from build123d import *

# Parameters (mm, degrees)
SKETCH1_R           = 4.6
SKETCH1_R_2         = 3
BOSS_EXTRUDE1_DEPTH = 6.6
SKETCH2_R           = 4.1
BOSS_EXTRUDE2_DEPTH = 6
CHAMFER2_SIZE       = 0.5
CHAMFER3_SIZE       = 0.4
CHAMFER4_SIZE       = 0.4
CHAMFER4_SIZE2      = 0.8
CHAMFER5_SIZE       = 0.4


with BuildPart() as part:
    # Sketch1 → Boss-Extrude1 (new body)
    with BuildSketch(Plane.XY):
        Circle(SKETCH1_R)
        Circle(SKETCH1_R_2, mode=Mode.SUBTRACT)
    extrude(amount=BOSS_EXTRUDE1_DEPTH)

    # Sketch2 → Boss-Extrude2 (add)
    with BuildSketch(Plane.XY.offset(6.6)):
        Circle(SKETCH2_R)
        with BuildLine():
            Line((1.6, -1.920937271), (1.6, 1.920937271))
            ThreePointArc((1.6, 1.920937271), (-2.5, 0), (1.6, -1.920937271))
        make_face(mode=Mode.SUBTRACT)
    extrude(amount=BOSS_EXTRUDE2_DEPTH)

    # Chamfer2
    chamfer2_edges = [part.edges().sort_by_distance(p)[0] for p in [
        (-4.6, 0, 6.6),
    ]]
    chamfer(chamfer2_edges, length=CHAMFER2_SIZE - 0.0001)  # a hair under: the kernel refuses the full size

    # Chamfer3
    chamfer3_edges = [part.edges().sort_by_distance(p)[0] for p in [
        (-2.5, 0, 12.6),
        (1.6, 0, 12.6),
        (-3, 0, 0),
    ]]
    chamfer(chamfer3_edges, length=CHAMFER3_SIZE)

    # Chamfer4
    chamfer4_edges = [part.edges().sort_by_distance(p)[0] for p in [
        (-3, 0, 6.6),
    ]]
    chamfer4_side = [part.faces().sort_by_distance(p)[0] for p in [
        (-2.915147186, 0, 6.6),
    ]]
    chamfer(chamfer4_edges, length=CHAMFER4_SIZE, length2=CHAMFER4_SIZE2, reference=chamfer4_side[0])

    # Chamfer5
    chamfer5_edges = [part.edges().sort_by_distance(p)[0] for p in [
        (-4.1, 0, 12.6),
        (-4.6, 0, 0),
    ]]
    chamfer(chamfer5_edges, length=CHAMFER5_SIZE)


solid = part.part
Work out the finished part from the listing and answer in its coordinate system (mm). A direction names the side the tool comes from. Give positions to 0.01 mm unless a question says otherwise; leave off trailing zeros. Order: outer loops, then holes, each group sorted by start corner. A loop starts at its lowest first (then second) coordinate and runs counter-clockwise, first axis right, second up. Notation, with made-up numbers: (15, 77) -> (54, 77) arc R7 ccw to (54, 81) -> close; hole circle Ø1 at (-21, 17). An arc over 180 degrees is marked (long way). One line per item, written item: value.
Item 1: Straight lines are drawn through the part: probe 1 along Y at (x, z) = (0, 2.9); probe 2 along Y at (x, z) = (0, 9.95); probe 3 along X at (y, z) = (0.5, 4.75). For each, find the intervals that lie inside material, in ascending order.
Answer sheet:
probe 1: -4.6 to -3, 3 to 4.6
probe 2: -4.1 to -2.5, 2.5 to 4.1
probe 3: -4.57 to -2.96, 2.96 to 4.57
Item 2: Find section C-C, the plane z = 2.25. Give the vertices of the cut face in (x, y), plus the area to 3 significant figures.
Answer sheet:
outline: circle Ø9.2 at (0, 0); hole circle Ø6 at (0, 0)
area: 38.2 mm²
Item 3: Flat-ended cylindrical pins translate along their axes: P1, Ø1.6, axis at x = 0, y = -1, coming from the -Z side; P2, Ø4, axis at y = -0.5, z = 8.5, coming from the -X side; P3, Ø2, axis at x = -3, z = 8, coming from the -Y side. Find the tip coordinate at first contact, or state that the pin passes through.
Answer sheet:
P1: through
P2: x = -4.18
P3: y = -3.58
Item 4: Determine the mould class of faces 1 (the cylindrical face through (-0.534, 4.065, 9.361)), 2 (the flat face through (2, -3, 0)), 3 (the flat face through (1.6, 0, 9)) for opening direction Y: released by +Y, released by -Y, zero draft, split by the parting line, or undercut.
Answer sheet:
face 1: split by the parting line
face 2: zero draft
face 3: undercut
Item 5: A tool of negligible diameter and unlimited length cuts with its end or side. For faces 4 (the cylindrical face through (-3, 0, 3)), 5 (the cylindrical face through (-2.5, 0.1, 9.4)), from which of +Z, -Z, +X, -X, +Y, -Y can it reach the whole face along a straight path? Write none if from no direction.
Answer sheet:
face 4: -Z
face 5: +Z, -Z
